Geometry: final body of the model. Coordinates: model frame, mm. Face numbers are marked on the shaded views. Coordinates: 2 decimals unless noted, no trailing zeros. Write each loop counter-clockwise with the first axis right and the second up, starting at its lowest first coordinate (ties: lowest second). Pieces come first, ordered by that corner, then holes.
from build123d import *

# Parameters (mm, degrees)
SKIZZE1_W                       = 80
SKIZZE1_H                       = 80
SKIZZE1_R                       = 2.5
AUFSATZ_LINEAR_AUSTRAGEN1_DEPTH = 6
M4_GEWINDEBOHRUNG2_D            = 3.3
M4_GEWINDEBOHRUNG2_DEPTH        = 11.5
M4_GEWINDEBOHRUNG2_TIP          = 0.991420021


with BuildPart() as part:
    # Skizze1 → Aufsatz-Linear austragen1 (new body)
    with BuildSketch(Plane.XY):
        Rectangle(SKIZZE1_W, SKIZZE1_H)
        Circle(SKIZZE1_R, mode=Mode.SUBTRACT)
    extrude(amount=AUFSATZ_LINEAR_AUSTRAGEN1_DEPTH)

    # M4 Gewindebohrung2
    with Locations(Plane(origin=(0, 0, 0), x_dir=(-1, 0, 0), z_dir=(0, 0, -1))):
        with Locations((35, 35), (35, -35), (-35, -35), (-35, 35)):
            Hole(M4_GEWINDEBOHRUNG2_D / 2, depth=M4_GEWINDEBOHRUNG2_DEPTH)
            with Locations((0, 0, -(M4_GEWINDEBOHRUNG2_DEPTH + M4_GEWINDEBOHRUNG2_TIP / 2))):  # 118° drill point
                Cone(0, M4_GEWINDEBOHRUNG2_D / 2, M4_GEWINDEBOHRUNG2_TIP, mode=Mode.SUBTRACT)

    # Skizze8 → Formsenkung für M8 Linsensenkschraube1 (revolve, cut)
    with BuildSketch(Plane.YZ):
        Polygon((0, 0), (0, 6), (4.5, 6), (4.5, 4.15), (8.65, 0), align=None)
    revolve(axis=Axis((0, 0, -6.35), (0, 0, 1)), mode=Mode.SUBTRACT)


solid = part.part
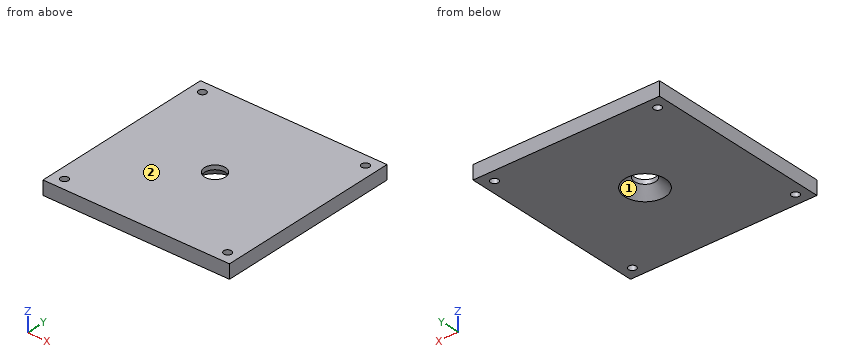
Item 1: Section D-D, the plane y = 0. Output: boundary loops of the cut face in (x, z), plus the area to 3 significant figures.
Derived:
outline: (-40, 0) - (-8.65, 0) - (-4.5, 4.15) - (-4.5, 6) - (-40, 6) - close; (4.5, 4.15) - (8.65, 0) - (40, 0) - (40, 6) - (4.5, 6) - close
area: 409 mm2
Item 2: Section A-A, the plane y = 35. Output: boundary loops of the cut face in (x, z), plus the area to 3 significant figures.
Derived:
outline: (-40, 0) - (-36.65, 0) - (-36.65, 6) - (-40, 6) - close; (-33.35, 0) - (33.35, 0) - (33.35, 6) - (-33.35, 6) - close; (36.65, 0) - (40, 0) - (40, 6) - (36.65, 6) - close
area: 440 mm2
Item 3: Section B-B, the plane z = 1.25. Output: boundary loops of the cut face in (x, y), plus the area to 3 significant figures.
Derived:
outline: (-40, -40) - (40, -40) - (40, 40) - (-40, 40) - close; hole circle Ø3.3 at (-35, -35); hole circle Ø3.3 at (-35, 35); hole circle Ø14.8 at (0, 0); hole circle Ø3.3 at (35, -35); hole circle Ø3.3 at (35, 35)
area: 6,190 mm2
Item 4: Pin query (flat end, axial travel): pin 1 (11.5 mm diameter, centred on x = 0, y = 0, fed in from -Z). Return the tip coordinate at first contact, or that it passes through.
Derived:
pin 1: stops at z = 2.9
Item 5: Pull-direction query (Y, two-part tool) for the marked faces 1 and 2; classes: released by +Y, released by -Y, zero draft, split by the parting line, or undercut.
Derived:
face 1: undercut
face 2: zero draft
Item 6: Material intervals for probe 1 along Y at (x, z) = (-35, 3.8); probe 2 along X at (y, z) = (0, 5.5); probe 3 along Y at (x, z) = (34, 5.5), sorted ascending.
Derived:
probe 1: y = -40 to -36.65, -33.35 to 33.35, 36.65 to 40
probe 2: x = -40 to -4.5, 4.5 to 40
probe 3: y = -40 to -36.31, -33.69 to 33.69, 36.31 to 40
